Autodesk Inventor part; units mm, degrees
ref_plane "作業平面1" through (14, 0, 0) normal (1, 0, 0) x (0, 1, 0)
ref_plane "作業平面2" through (-14, 0, 0) normal (1, 0, 0) x (0, 1, 0)
ref_plane "作業平面3" through (0, 7.5, 0) normal (0, 1, 0) x (-1, 0, 0)
sketch "スケッチ1" plane through (0, 0, 0) normal (0, 0, 1) x (1, 0, 0)
  circle A0 centre (0, 0) radius 7.5
  dimension "d0" = 15
extrude "押し出し1" add sketch "スケッチ1" along normal blind 40
sketch "スケッチ2" plane through (0, 0, 0) normal (0, 0, -1) x (-1, 0, 0)
  arc A0 (-2.9394, 3) -> (2.9394, 3) centre (0, 0) ccw
  line L0 (-2.9394, 3) -> (2.9394, 3)
  point P0 (-3.1305, 2.8)
  dimension "d3" = 4.2
  dimension "d4" = 3
extrude "押し出し2" cut sketch "スケッチ2" against normal blind 30
ref_plane "作業平面1" through (14, 0, 0) normal (1, 0, 0) x (0, 1, 0)
ref_plane "作業平面2" through (-14, 0, 0) normal (1, 0, 0) x (0, 1, 0)
ref_plane "作業平面3" through (0, 7.5, 0) normal (0, 1, 0) x (-1, 0, 0)
ref_plane "作業平面4" through (0, -7.5, 0) normal (0, 1, 0) x (-1, 0, 0)
sketch "スケッチ7" plane through (0, 7.5, 0) normal (0, 1, 0) x (-1, 0, 0)
  circle A0 centre (0, 12.5) radius 1.7
  point P0 (0, 0)
  dimension "d35" = 3.4
  dimension "d36" = 12.5
extrude "押し出し7" cut sketch "スケッチ7" against normal through all
sketch "スケッチ8" plane through (0, 7.5, 0) normal (0, 1, 0) x (-1, 0, 0)
  circle A0 centre (0, 12.5) radius 3.25
  point P0 (0, 0)
  dimension "d39" = 6.5
  dimension "d40" = 12.5
sketch "スケッチ9" plane through (0, -7.5, 0) normal (0, 1, 0) x (-1, 0, 0)
  circle A0 centre (0, 12.5) radius 3.25
  point P0 (0, 0)
  dimension "d41" = 6.5
  dimension "d42" = 12.5
extrude "押し出し8" cut sketch "スケッチ8" against normal blind 1
extrude "押し出し9" cut sketch "スケッチ9" along normal blind 1
sketch "スケッチ10" plane through (0, 0, 40) normal (0, 0, 1) x (1, 0, 0)
  circle A0 centre (0, 0) radius 14
  dimension "d47" = 28
extrude "押し出し10" add sketch "スケッチ10" along normal blind 10
ref_plane "作業平面5" through (0, 14, 0) normal (0, 1, 0) x (-1, 0, 0)
ref_plane "作業平面6" through (0, -14, 0) normal (0, 1, 0) x (-1, 0, 0)
sketch "スケッチ11" plane through (0, 14, 0) normal (0, 1, 0) x (-1, 0, 0)
  circle A0 centre (0, 45) radius 1.5
  line L0 (14, 50) -> (-14, 50)
  point P0 (0, 0)
  dimension "d52" = 3
  dimension "d53" = 5
sketch "スケッチ12" plane through (0, -14, 0) normal (0, 1, 0) x (-1, 0, 0)
  circle A0 centre (0, 45) radius 1.5
  line L0 (14, 50) -> (-14, 50)
  point P0 (0, 0)
  dimension "d54" = 3
  dimension "d55" = 5
sketch "スケッチ13" plane through (-14, 0, 0) normal (1, 0, 0) x (0, 1, 0)
  circle A0 centre (0, 45) radius 1.5
  line L0 (14, 50) -> (-14, 50)
  point P0 (0, 0)
  dimension "d56" = 3
  dimension "d57" = 5
sketch "スケッチ14" plane through (14, 0, 0) normal (1, 0, 0) x (0, 1, 0)
  circle A0 centre (0, 45) radius 1.5
  line L0 (14, 50) -> (-14, 50)
  point P0 (0, 0)
  dimension "d58" = 3
  dimension "d59" = 5
extrude "押し出し11" cut sketch "スケッチ11" against normal blind 10
extrude "押し出し12" cut sketch "スケッチ12" along normal blind 10
extrude "押し出し13" cut sketch "スケッチ14" against normal blind 10
extrude "押し出し14" cut sketch "スケッチ13" along normal blind 10
thread "ねじ5"
thread "ねじ6"
thread "ねじ7"
thread "ねじ8"
sketch "スケッチ15" plane through (0, 0, 50) normal (0, 0, 1) x (1, 0, 0)
  circle A0 centre (7.5, 7.5) radius 1.7
  circle A1 centre (-7.5, 7.5) radius 1.7
  circle A2 centre (-7.5, -7.5) radius 1.7
  circle A3 centre (7.5, -7.5) radius 1.7
  point P0 (0, 0)
  dimension "d76" = 3.4
  dimension "d77" = 7.5
  dimension "d78" = 7.5
  dimension "d81" = 360
extrude "押し出し15" cut sketch "スケッチ15" against normal through all
properties part number "rotary_transfer_shaft_5_1" material "ステンレス鋼"
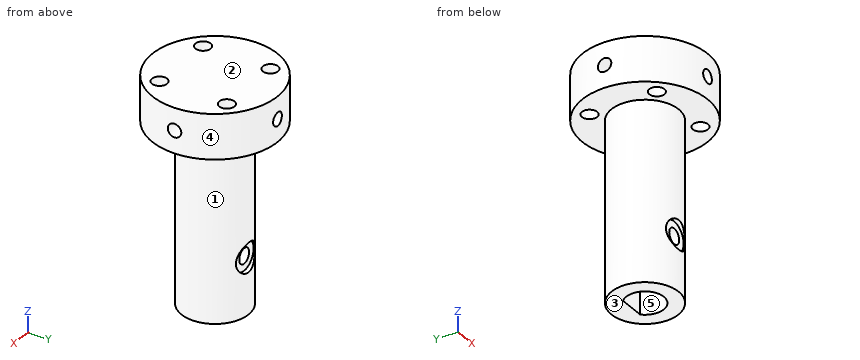
Verification items for the finished model (mm, model axes). Face numbers are marked on the shaded views. A direction names the side the tool comes from. Round coordinates to 2 decimals unless told otherwise and drop trailing zeros. Order: outer loops, then holes, each group sorted by start corner. A loop starts at its lowest first (then second) coordinate and runs counter-clockwise, first axis right, second up. Notation, with made-up numbers: (32, 28.5) - (72, 28.5) arc R32 cw to (72, 61.5) - close; hole circle Ø5 at (11.25, 22.25). An arc over 180 degrees is marked (long way). Use CSV: the item, a comma, the result in double quotes. Start each with the question number.
1) Section check D-D, the plane x = 0. State how many separate pieces and enclosed holes the cut face has, plus the area to 3 significant figures.
2) Section check B-B, the plane x = -8.25. Record the cut outline in (y, z).
3) Access from +Z, -Z, +X, -X, +Y, -Y to the whole of each face (thin tool, end or side, straight path). Record for the marked faces 1 and 2.
4) Thickness scan on L1, parallel to Z at x = 0, y = 4.1; L2, parallel to Y at x = 7.5, z = 45.75; L3, parallel to Z at x = 9.75, y = 0. Record the ranges inside material, lowest first.
5) Section check C-C, the plane y = 5. Record the cut outline in (x, z).
6) Section check A-A, the plane z = 41. Record the cut outline in (x, y).
7) Go/stop test with flat-tipped pins: P1, Ø0.9, axis at y = -0.5, z = 44.5, coming from the +X side; P2, Ø2.5, axis at x = 0, z = 45, coming from the +Y side; P3, Ø2, axis at y = -8.5, z = 43.5, coming from the -X side; P4, Ø2.5, axis at x = -7.5, y = 7.5, coming from the +Z side. Record where each tip stops, or that it passes through.
8) Mould release check, pull along Y, two halves, no side actions. Record for the marked faces 3, 4 and 5: +Y half, -Y half, draft (parallel to the pull), parting line (faces both ways), or undercut.
Answers:
1,separate pieces,"3"
1,enclosed holes,"0"
1,area,"571 mm²"
2,outline,"(-11.31, 40) - (-9.03, 40) - (-9.03, 50) - (-11.31, 50) - close; (-5.97, 40) - (5.97, 40) - (5.97, 50) - (-5.97, 50) - close; (9.03, 40) - (11.31, 40) - (11.31, 50) - (9.03, 50) - close; hole circle Ø3 at (0, 45)"
3,face 1,"-Z"
3,face 2,"+Z, +X, -X, +Y, -Y"
4,L1,"z = 0 to 10.8, 14.2 to 43.5, 46.5 to 50"
4,L2,"y = -11.82 to -9.2, -5.8 to -1.3, 1.3 to 5.8, 9.2 to 11.82"
4,L3,"z = 40 to 43.5, 46.5 to 50"
5,outline,"(-13.08, 40) - (-5.59, 40) - (-5.59, 0) - (5.59, 0) - (5.59, 40) - (13.08, 40) - (13.08, 50) - (-13.08, 50) - close; hole circle Ø3.4 at (0, 12.5); hole circle Ø3 at (0, 45)"
6,outline,"circle Ø28 at (0, 0); hole circle Ø3.4 at (-7.5, -7.5); hole circle Ø3.4 at (-7.5, 7.5); hole circle Ø3.4 at (7.5, -7.5); hole circle Ø3.4 at (7.5, 7.5)"
7,P1,"stops at x = 4"
7,P2,"stops at y = 4"
7,P3,"stops at x = -11.82"
7,P4,"passes through"
8,face 3,"draft"
8,face 4,"parting line"
8,face 5,"undercut"
